Read the model definition and answer for the solid it produces. Units are mm, in the model's axes. A direction names the side the tool comes from. Round coordinates to 2 decimals unless told otherwise and drop trailing zeros. Order: outer loops, then holes, each group sorted by start corner. A loop starts at its lowest first (then second) coordinate and runs counter-clockwise, first axis right, second up. Notation, with made-up numbers: (46.5, 74.5) -> (87.5, 74.5) arc R13 ccw to (87.5, 92.5) -> close; hole circle Ø5 at (77, 35). An arc over 180 degrees is marked (long way). Use a Markdown table: item, result. Add a question column.
1. Section B-B, the plane y = 17.75 is taken. Give the vertices of the cut face in (x, z) (3 decimals), then the cut area to 3 significant figures.
2. Section C-C, the plane z = 14 is taken. Give the vertices of the cut face in (x, y).
3. Consider L1, parallel to X at y = 24.8, z = 0 (3 decimals); L2, parallel to Y at x = -30, z = -9; L3, parallel to Z at x = 8, y = 20.5. Determine where each line is inside the solid, lowest interval first. Write a range as [from, to].
4. The mould has two halves that part along Z. Classify faces 5 (the face through (7, 24, -2)), 6 (the face through (0, 23, 7.2)), 7 (the face through (36.99, 2.46, -37.15)): +Z half, -Z half, draft (parallel to the pull), parting line (faces both ways), or undercut.
5. For faces 1 (the face through (-22.496, 12.395, -0.378)), 2 (the face through (0, 2, -40)), 3 (the face through (-9.69, 11.83, 0.18)), 4 (the face through (0, 23, -7.2)), determine the directions among +Z, -Z, +X, -X, +Y, -Y from which every point of the face is accessible in a straight line to the end or side of a thin tool.
6. Section D-D, the plane x = 17 is taken. Give the vertices of the cut face in (y, z), then the cut area to 3 significant figures.
7. Given pin 1 (3 mm diameter, centred on x = -1, y = 24, fed in from +Z); pin 2 (1.5 mm diameter, centred on x = 12.5, y = 11.5, fed in from +Z); pin 3 (3.5 mm diameter, centred on x = -5.595, z = 0, fed in from -Y); pin 4 (4 mm diameter, centred on x = -6.5, z = 1.5, fed in from -Y), each flat-ended and moving along its own axis, determine where each tip first touches the part or whether it passes through.
8. Section A-A, the plane z = 0 is taken. Give the vertices of the cut face in (x, y) (3 decimals).
```python
from build123d import *

# Parameters (mm, degrees)
BOSS_EXTRUDE1_DEPTH = 5
BOSS_EXTRUDE2_DEPTH = 15
BOSS_EXTRUDE3_DEPTH = 6
SKETCH6_R           = 2.2
CUT_EXTRUDE1_DEPTH  = 27
SKETCH7_R           = 4.1
CUT_EXTRUDE2_DEPTH  = 24


with BuildPart() as part:
    # Sketch1 → Boss-Extrude1 (new body)
    with BuildSketch(Plane(origin=(0, 0, 0), x_dir=(1, 0, 0), z_dir=(0, 1, 0))):
        with BuildLine():
            Line((30, -40), (-30, -40))
            ThreePointArc((-30, -40), (-37.071067812, -37.071067812), (-40, -30))
            Line((-40, -30), (-40, 30))
            ThreePointArc((-40, 30), (-37.071067812, 37.071067812), (-30, 40))
            Line((-30, 40), (30, 40))
            ThreePointArc((30, 40), (37.071067812, 37.071067812), (40, 30))
            Line((40, 30), (40, -30))
            ThreePointArc((40, -30), (37.071067812, -37.071067812), (30, -40))
        make_face()
    extrude(amount=BOSS_EXTRUDE1_DEPTH)

    # Sketch4 → Boss-Extrude2 (add)
    with BuildSketch(Plane(origin=(0, 5, 0), x_dir=(1, 0, 0), z_dir=(0, 1, 0))):
        with BuildLine():
            Line((-5.29954084, -17.20045916), (5.29954084, -17.20045916))
            ThreePointArc((5.29954084, -17.20045916), (22.5, 0), (5.29954084, 17.20045916))
            Line((5.29954084, 17.20045916), (-5.29954084, 17.20045916))
            ThreePointArc((-5.29954084, 17.20045916), (-22.5, 0), (-5.29954084, -17.20045916))
        make_face()
    extrude(amount=BOSS_EXTRUDE2_DEPTH)

    # Sketch5 → Boss-Extrude3 (add)
    with BuildSketch(Plane(origin=(0, 20, 0), x_dir=(1, 0, 0), z_dir=(0, 1, 0))):
        with BuildLine():
            Line((-5.29954084, -7.20045916), (5.29954084, -7.20045916))
            ThreePointArc((5.29954084, -7.20045916), (12.5, 0), (5.29954084, 7.20045916))
            Line((5.29954084, 7.20045916), (-5.29954084, 7.20045916))
            ThreePointArc((-5.29954084, 7.20045916), (-12.5, 0), (-5.29954084, -7.20045916))
        make_face()
    extrude(amount=BOSS_EXTRUDE3_DEPTH)

    # Sketch6 → Cut-Extrude1 (cut)
    with BuildSketch(Plane(origin=(0, 26, 0), x_dir=(1, 0, 0), z_dir=(0, 1, 0))):
        with Locations((-5.595, 0)):
            Circle(SKETCH6_R)
        with Locations((5.595, 0)):
            Circle(SKETCH6_R)
    extrude(amount=-CUT_EXTRUDE1_DEPTH, mode=Mode.SUBTRACT)

    # Sketch7 → Cut-Extrude2 (cut)
    with BuildSketch(Plane.XZ):
        with Locations((5.595, 0)):
            Circle(SKETCH7_R)
        with Locations((-5.595, 0)):
            Circle(SKETCH7_R)
    extrude(amount=-CUT_EXTRUDE2_DEPTH, mode=Mode.SUBTRACT)


solid = part.part
```
Verdict:
| question | item | result |
|---|---|---|
| 1 | outline | (-5.3, -17.2) -> (5.3, -17.2) arc R17.2 ccw to (5.3, 17.2) -> (-5.3, 17.2) arc R17.2 ccw to start; hole circle Ø8.2 at (-5.595, 0); hole circle Ø8.2 at (5.595, 0) |
| 1 | area | 1,190 mm2 |
| 2 | outline | (-40, 0) -> (40, 0) -> (40, 5) -> (15.29, 5) -> (15.29, 20) -> (-15.29, 20) -> (-15.29, 5) -> (-40, 5) -> close |
| 3 | L1 | x = [-12.5, -7.795], [-3.395, 3.395], [7.795, 12.5] |
| 3 | L2 | y = [0, 5] |
| 3 | L3 | z = [-6.67, -3.32], [3.32, 6.67] |
| 4 | face 5 | undercut |
| 4 | face 6 | +Z half |
| 4 | face 7 | -Z half |
| 5 | face 1 | -X, +Y |
| 5 | face 2 | -Z, +X, -X, +Y, -Y |
| 5 | face 3 | -Y |
| 5 | face 4 | -Z, +X, -X, +Y |
| 6 | outline | (0, -40) -> (5, -40) -> (5, -12.61) -> (20, -12.61) -> (20, 12.61) -> (5, 12.61) -> (5, 40) -> (0, 40) -> close |
| 6 | area | 778 mm2 |
| 7 | pin 1 | stops at z = 7.2 |
| 7 | pin 2 | stops at z = 15.95 |
| 7 | pin 3 | passes through |
| 7 | pin 4 | stops at y = 24 |
| 8 | outline | (-40, 0) -> (-9.695, 0) -> (-9.695, 24) -> (-7.795, 24) -> (-7.795, 26) -> (-12.5, 26) -> (-12.5, 20) -> (-22.5, 20) -> (-22.5, 5) -> (-40, 5) -> close; (-3.395, 24) -> (-1.495, 24) -> (-1.495, 0) -> (1.495, 0) -> (1.495, 24) -> (3.395, 24) -> (3.395, 26) -> (-3.395, 26) -> close; (7.795, 24) -> (9.695, 24) -> (9.695, 0) -> (40, 0) -> (40, 5) -> (22.5, 5) -> (22.5, 20) -> (12.5, 20) -> (12.5, 26) -> (7.795, 26) -> close |
